from build123d import *

# Parameters (mm, degrees)
F1_DEPTH = 3.75
F2_R     = 3.70839
F4_DEPTH = 3.9243
F5_R     = 2.413
F6_DEPTH = 3.75
F7_R     = 3.0607
F8_DEPTH = 0.5


# Not quite as in the source:
# - a fillet or chamfer is up to 0.001 mm smaller than in the source, because OpenCascade refuses the exact size
# - a length typed as a fraction of an inch, garbled in the dataset ("3 / 203.2 mm" for 3/8 in), is restored


with BuildPart() as f1:
    # F0 (on Front) → F1 (new body)
    with BuildSketch(Plane.XZ):
        Polygon((3.7084, 11.5824), (-19.4564, 11.5824), (-19.4564, 4.1656), (-3.7084, 4.1656), (-3.7084, -11.5824), (19.4564, -11.5824), (19.4564, -4.1656), (3.7084, -4.1656), align=None)
    extrude(amount=F1_DEPTH)

    # F2 (radius 3.7084 in the source; OpenCascade refuses exactly that, so slightly less here)
    f2_edges = [f1.edges().sort_by_distance(p)[0] for p in [
        (-19.4564, -1.875, 11.5824),
        (3.7084, -1.875, 11.5824),
        (19.4564, -1.875, -4.1656),
        (19.4564, -1.875, -11.5824),
        (-3.7084, -1.875, -11.5824),
        (-19.4564, -1.875, 4.1656),
    ]]
    fillet(f2_edges, radius=F2_R)

    # F3 (on face) → F4 (cut)
    with BuildSketch(Plane.XZ.offset(3.75)):
        with BuildLine():
            Line((-9.9491970991, 10.9474), (-13.6728029009, 10.9474))
            ThreePointArc((-13.6728029009, 10.9474), (-12.0396, 7.874), (-13.6728029009, 4.8006))
            Line((-13.6728029009, 4.8006), (-9.9491970991, 4.8006))
            ThreePointArc((-9.9491970991, 4.8006), (-11.5824, 7.874), (-9.9491970991, 10.9474))
        make_face()
        with BuildLine():
            Line((-2.0751970991, 10.9474), (-5.7988029009, 10.9474))
            ThreePointArc((-5.7988029009, 10.9474), (-4.5992563854, 9.6141967759), (-4.1656, 7.874))
            ThreePointArc((-4.1656, 7.874), (-3.937, 7.6454), (-3.7084, 7.874))
            ThreePointArc((-3.7084, 7.874), (-3.2747436146, 9.6141967759), (-2.0751970991, 10.9474))
        make_face()
        with BuildLine():
            Line((3.0734, 2.0751970991), (3.0734, 5.7988029009))
            ThreePointArc((3.0734, 5.7988029009), (1.7401967759, 4.5992563854), (0, 4.1656))
            ThreePointArc((0, 4.1656), (-0.2286, 3.937), (0, 3.7084))
            ThreePointArc((0, 3.7084), (1.7401967759, 3.2747436146), (3.0734, 2.0751970991))
        make_face()
        with BuildLine():
            ThreePointArc((0, -3.7084), (-1.7401967759, -3.2747436146), (-3.0734, -2.0751970991))
            Line((-3.0734, -2.0751970991), (-3.0734, -5.7988029009))
            ThreePointArc((-3.0734, -5.7988029009), (-1.7401967759, -4.5992563854), (0, -4.1656))
            ThreePointArc((0, -4.1656), (0.2286, -3.937), (0, -3.7084))
        make_face()
        with BuildLine():
            ThreePointArc((3.7084, -7.874), (3.2747436146, -9.6141967759), (2.0751970991, -10.9474))
            Line((2.0751970991, -10.9474), (5.7988029009, -10.9474))
            ThreePointArc((5.7988029009, -10.9474), (4.5992563854, -9.6141967759), (4.1656, -7.874))
            ThreePointArc((4.1656, -7.874), (3.937, -7.6454), (3.7084, -7.874))
        make_face()
        with BuildLine():
            ThreePointArc((9.9491970991, -4.8006), (11.5824, -7.874), (9.9491970991, -10.9474))
            Line((9.9491970991, -10.9474), (13.6728029009, -10.9474))
            ThreePointArc((13.6728029009, -10.9474), (12.0396, -7.874), (13.6728029009, -4.8006))
            Line((13.6728029009, -4.8006), (9.9491970991, -4.8006))
        make_face()
    extrude(amount=-F4_DEPTH, mode=Mode.SUBTRACT)

    # F5 (on face) → F6 (cut, through all)
    with BuildSketch(Plane.XZ.offset(3.75)):
        with Locations((-15.748, 7.874)):
            Circle(F5_R)
        with Locations((0, 7.874)):
            Circle(F5_R)
        with Locations((0, -7.874)):
            Circle(F5_R)
        with Locations((15.748, -7.874)):
            Circle(F5_R)
        with Locations((-7.874, 7.874)):
            Circle(F5_R)
        Circle(F5_R)
        with Locations((7.874, -7.874)):
            Circle(F5_R)
    extrude(amount=-F6_DEPTH, mode=Mode.SUBTRACT)

    # F7 (on face) → F8 (cut)
    with BuildSketch(Plane.XZ.offset(3.75)):
        with Locations((-15.748, 7.874)):
            Circle(F7_R)
        with Locations((-7.874, 7.874)):
            Circle(F7_R)
        with Locations((0, 7.874)):
            Circle(F7_R)
        Circle(F7_R)
        with Locations((0, -7.874)):
            Circle(F7_R)
        with Locations((7.874, -7.874)):
            Circle(F7_R)
        with Locations((15.748, -7.874)):
            Circle(F7_R)
    extrude(amount=-F8_DEPTH, mode=Mode.SUBTRACT)

    # F9: F1 across plane


with BuildPart() as f1_1:
    add(f1.part)
    add(f1.part.mirror(Plane.XZ))


solid = f1_1.part
The model under review builds one solid part; all positions refer to its coordinate system, in mm. A direction names the side the tool comes from. Round coordinates to 2 decimals unless told otherwise and drop trailing zeros. Order: outer loops, then holes, each group sorted by start corner. A loop starts at its lowest first (then second) coordinate and runs counter-clockwise, first axis right, second up. Notation, with made-up numbers: (46, 9) -> (73, 9) arc R27 ccw to (73, 44) -> close; hole circle Ø7 at (24.25, 8.25). An arc over 180 degrees is marked (long way). Write item = value, one per line. Start each with the question number.
Item 1: Mouldability with a two-part tool opening along X and no side actions: class faces 1 (the face through (-2.65, 0.05, -10.47)), 2 (the face through (2.593, 0.053, 10.525)), 3 (the face through (12.69, -3.5, -7.74)) as released by +X, released by -X, zero draft, split by the parting line, or undercut.
Item 2: For faces 4 (the face through (18.4, 0.05, -5.28)), 5 (the face through (16, 3.25, -5)), 6 (the face through (8, -3.25, -5)), list the 3-axis set-ups (+Z, -Z, +X, -X, +Y, -Y) from which the entire face can be reached by the end or side of a thin tool; tool diameter is ignored.
Item 3: Consider section B-B on x = 7.5. Write out the cut boundary in (y, z).
Item 4: Clearance check with flat-ended pins moving along their axes: pin 1 Ø1.8 at (x, z) = (-1.5, -1) entering from -Y; pin 2 Ø4.5 at (x, z) = (0, -7.874) entering from -Y; pin 3 Ø1.8 at (x, z) = (-1, -6.5) entering from +Y; pin 4 Ø2 at (x, y) = (7.5, 1.5) entering from +Z. State where each tip first meets the part, or that it passes through.
Item 5: For line 1 along Z through (x, y) = (2, 0); line 2 along Z through (x, y) = (10.5, -2.75); line 3 along Z through (x, y) = (-1.5, -2.75), list the stretches that pass through material, from the lowest coordinate up.
Item 6: Consider section A-A on z = 0. Write out the cut boundary in (x, y).
Item 7: Consider section C-C on y = -1. Count the separate pieces of the cut face and the enclosed holes in it, plus the area to 3 significant figures.
Conclusion:
q1.face_1 = released by -X
q1.face_2 = released by +X
q1.face_3 = undercut
q2.face_4 = +Z, +X, +Y, -Y
q2.face_5 = +Y
q2.face_6 = -Y
q3.outline = (-3.75, -11.58) -> (3.75, -11.58) -> (3.75, -10.91) -> (3.25, -10.91) -> (3.25, -10.26) -> (-3.25, -10.26) -> (-3.25, -10.91) -> (-3.75, -10.91) -> close; (-3.75, -4.84) -> (-3.25, -4.84) -> (-3.25, -5.49) -> (3.25, -5.49) -> (3.25, -4.84) -> (3.75, -4.84) -> (3.75, -4.17) -> (-3.75, -4.17) -> close
q4.pin_1 = -3.25
q4.pin_2 = through
q4.pin_3 = 3.25
q4.pin_4 = -4.17
q5.line_1 = -11.58 to -9.22, -6.52 to -1.35, 1.35 to 3.12, 4.75 to 6.52, 9.22 to 11
q5.line_2 = -11.58 to -10.95, -10.49 to -5.26, -4.8 to -4.17
q5.line_3 = -11.27 to -9.76, -5.98 to -4.48, -3.39 to -1.89, 1.89 to 5.98, 9.76 to 11.58
q6.outline = (-3.71, -3.75) -> (-3.06, -3.75) -> (-3.06, -3.25) -> (-2.41, -3.25) -> (-2.41, 3.25) -> (-3.06, 3.25) -> (-3.06, 3.75) -> (-3.71, 3.75) -> close; (2.41, -3.25) -> (3.06, -3.25) -> (3.06, -3.75) -> (3.71, -3.75) -> (3.71, 3.75) -> (3.06, 3.75) -> (3.06, 3.25) -> (2.41, 3.25) -> close
q7.separate_pieces = 1
q7.enclosed_holes = 13
q7.area = 224 mm2
